from build123d import *

# Parameters (mm, degrees)
F0_R     = 3.25
F0_W     = 3.3
F0_H     = 6.5
F1_DEPTH = 0.2
F2_R     = 5
F3_W     = 24.7
F3_H     = 0.02
F4_DEPTH = 0.02
F5_R     = 1


with BuildPart() as f1:
    # F0 (on Top) → F1 (new body)
    with BuildSketch(Plane.XY):
        with BuildLine():
            Line((13.2, 4.35), (-13.2, 4.35))
            add(Edge.make_bspline(
                [(-13.2, 4.35), (-20.78037737, -0.0910291662), (-13, -4.4647700118)],
                knots=[2.4980915448, 2.4980915448, 2.4980915448, 3.8050320878, 3.8050320878, 3.8050320878], degree=2, weights=[1, 0.7939788481, 1]))
            ThreePointArc((-13, -4.4647700118), (-11.3932239297, -6.7993510754), (-11.7365717654, -9.6125539381))
            ThreePointArc((-11.7365717654, -9.6125539381), (-12.1943796042, -10.8190157973), (-12.35, -12.1))
            Line((-12.35, -12.1), (-12.35, -22.8))
            ThreePointArc((-12.35, -22.8), (-10.7830212793, -26.5830212793), (-7, -28.15))
            Line((-7, -28.15), (7, -28.15))
            ThreePointArc((7, -28.15), (10.7830212793, -26.5830212793), (12.35, -22.8))
            Line((12.35, -22.8), (12.35, -12.1))
            ThreePointArc((12.35, -12.1), (12.1943796042, -10.8190157973), (11.7365717654, -9.6125539381))
            ThreePointArc((11.7365717654, -9.6125539381), (11.3932239297, -6.7993510754), (13, -4.4647700118))
            add(Edge.make_bspline(
                [(13, -4.4647700118), (20.78037737, -0.0910291662), (13.2, 4.35)],
                knots=[5.6197458729, 5.6197458729, 5.6197458729, 6.926686416, 6.926686416, 6.926686416], degree=2, weights=[1, 0.7939788481, 1]))
        make_face()
        with Locations((-7, -22.8)):
            Circle(F0_R, mode=Mode.SUBTRACT)
        with Locations((-7, -12.1)):
            Circle(F0_R, mode=Mode.SUBTRACT)
        with Locations((7, -22.8)):
            Circle(F0_R, mode=Mode.SUBTRACT)
        with Locations((0, -12.1)):
            Rectangle(F0_W, F0_H, mode=Mode.SUBTRACT)
        with Locations((7, -12.1)):
            Circle(F0_R, mode=Mode.SUBTRACT)
    extrude(amount=F1_DEPTH)

    # F2
    f2_edges = [f1.edges().sort_by_distance(p)[0] for p in [
        (13.2, 4.35, 0.1),
        (-13.2, 4.35, 0.1),
    ]]
    fillet(f2_edges, radius=F2_R)

    # F3 (on face) → F4 (cut)
    with BuildSketch(Plane(origin=(0, 0, 0), x_dir=(1, 0, 0), z_dir=(0, 0, -1))):
        with Locations((0, 17.45)):
            Rectangle(F3_W, F3_H)
    extrude(amount=-F4_DEPTH, mode=Mode.SUBTRACT)

    # F5
    f5_edges = [f1.edges().sort_by_distance(p)[0] for p in [
        (-1.65, -8.85, 0.1),
        (1.65, -8.85, 0.1),
        (-1.65, -15.35, 0.1),
        (1.65, -15.35, 0.1),
    ]]
    fillet(f5_edges, radius=F5_R)


solid = f1.part
Could you check a few things on this model? Use its own coordinates, in mm. Give positions to 0.01 mm unless a question says otherwise; leave off trailing zeros. Order: outer loops, then holes, each group sorted by start corner. A loop starts at its lowest first (then second) coordinate and runs counter-clockwise, first axis right, second up.
1. Suppose I cut it at C-C (y = -16.5). List the corners of the cut face in (x, z) for me, plus the area to 3 significant figures.
2. I need wall thicknesses on L1, parallel to Y at x = -7, z = 0.15; L2, parallel to X at y = -25, z = 0.1. Which ranges of each line are inside material? Lowest first, please.
3. Suppose I cut it at A-A (x = -7.5). Give the number of separate pieces and of enclosed holes in the cut face, plus the area to 3 significant figures.
Solved:
1. outline: (-12.35, 0) - (12.35, 0) - (12.35, 0.2) - (-12.35, 0.2) - close
1. area: 4.94 mm2
2. L1: y = -28.15 to -26.05, -19.55 to -15.35, -8.85 to 4.35
2. L2: x = -11.88 to -9.39, -4.61 to 4.61, 9.39 to 11.88
3. separate pieces: 3
3. enclosed holes: 0
3. area: 3.93 mm2
